Verification items for the finished model (mm, model axes). A direction names the side the tool comes from. Give positions to 0.01 mm unless a question says otherwise; leave off trailing zeros. Loops run counter-clockwise (first coordinate to the right, second up) from the corner with the lowest first, then second, coordinate; pieces in that order, holes last. Notation, with made-up numbers: (33.25, -11.75) - (80.25, -11.75) arc R15 ccw to (80.25, -6.75) - close; hole circle Ø4 at (-18, -12). An arc over 180 degrees is marked (long way). One line per item, written item: value. Start each with the question number.
1. Scan lines: L1, parallel to X at y = 16, z = -4; L2, parallel to Z at x = 0, y = 13; L3, parallel to Z at x = 31, y = 12.75. Record each from-to range of solid material in increasing order. Write a range as [from, to].
2. Mould release check, pull along X, two halves, no side actions. Record for faces 1 (the flat face through (-40, 13, 1)), 2 (the flat face through (8, 25.4, -1)), 3 (the flat face through (20.95, 13, 0)), 4 (the flat face through (-33.65, 13, 0)): pulls with the +X half, pulls with the -X half, needs draft (parallel to the pull), parting line crosses it, or undercut.
3. Gauge pin test, flat end, axial feed: pin 1 (1.1 mm diameter, centred on x = 0, z = 0, fed in from -Y). Record the tip position at first contact, or that the pin passes through.
4. Sectioned sample at B-B (x = 29.5). Record the cut outline in (y, z), plus the area to 3 significant figures.
5. Access from +Z, -Z, +X, -X, +Y, -Y to the whole of each face (thin tool, end or side, straight path). Record for faces 5 (the flat face through (-27, 13, -6.35)), 6 (the flat face through (-1, 13, 40)).
6. Sectioned sample at A-A (y = 19). Record the cut outline in (x, z).
from build123d import *

# Parameters (mm, degrees)
SKETCH1_W                                         = 80
SKETCH1_H                                         = 80
SKETCH1_W_2                                       = 12.7
SKETCH1_H_2                                       = 12.7
BOSS_EXTRUDE1_DEPTH                               = 25.4
CSK_FOR_0_FLAT_HEAD_MACHINE_SCREW_100_D           = 1.778
CSK_FOR_0_FLAT_HEAD_MACHINE_SCREW_100_CSINK_D     = 3.0226
CSK_FOR_0_FLAT_HEAD_MACHINE_SCREW_100_CSINK_ANGLE = 100


with BuildPart() as part:
    # Sketch1 → Boss-Extrude1 (new body)
    with BuildSketch(Plane(origin=(0, 0, 0), x_dir=(1, 0, 0), z_dir=(0, 1, 0))):
        Rectangle(SKETCH1_W, SKETCH1_H)
        with Locations((-27.3, 0)):
            Rectangle(SKETCH1_W_2, SKETCH1_H_2, mode=Mode.SUBTRACT)
        with Locations((27.3, 0)):
            Rectangle(SKETCH1_W_2, SKETCH1_H_2, mode=Mode.SUBTRACT)
    extrude(amount=BOSS_EXTRUDE1_DEPTH)

    # CSK for #0 Flat Head Machine Screw (100)1 (through all)
    with Locations(Plane(origin=(0, 25.4, 0), x_dir=(1, 0, 0), z_dir=(0, 1, 0))):
        with Locations((0, 0)):
            CounterSinkHole(CSK_FOR_0_FLAT_HEAD_MACHINE_SCREW_100_D / 2, CSK_FOR_0_FLAT_HEAD_MACHINE_SCREW_100_CSINK_D / 2, counter_sink_angle=CSK_FOR_0_FLAT_HEAD_MACHINE_SCREW_100_CSINK_ANGLE)


solid = part.part
Results are:
1. L1: x = [-40, -33.65], [-20.95, 20.95], [33.65, 40]
1. L2: z = [-40, -0.89], [0.89, 40]
1. L3: z = [-40, -6.35], [6.35, 40]
2. face 1: pulls with the -X half
2. face 2: needs draft
2. face 3: undercut
2. face 4: undercut
3. pin 1: passes through
4. outline: (0, -40) - (25.4, -40) - (25.4, -6.35) - (0, -6.35) - close; (0, 6.35) - (25.4, 6.35) - (25.4, 40) - (0, 40) - close
4. area: 1,710 mm^2
5. face 5: +Y, -Y
5. face 6: +Z, +X, -X, +Y, -Y
6. outline: (-40, -40) - (40, -40) - (40, 40) - (-40, 40) - close; hole (-33.65, -6.35) - (-20.95, -6.35) - (-20.95, 6.35) - (-33.65, 6.35) - close; hole circle Ø1.78 at (0, 0); hole (20.95, -6.35) - (33.65, -6.35) - (33.65, 6.35) - (20.95, 6.35) - close
